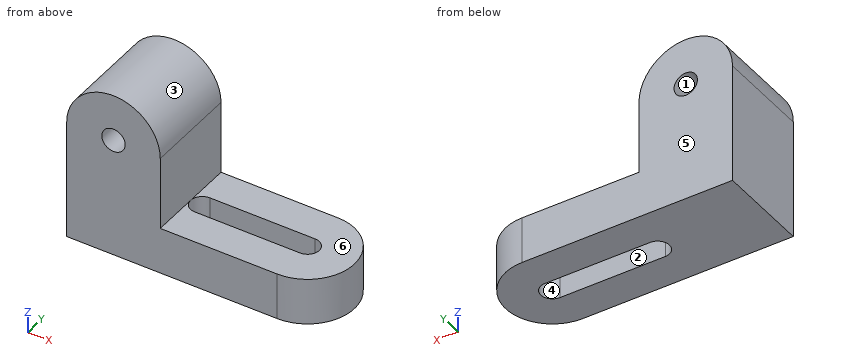
```python
from build123d import *

# Parameters (mm, degrees)
F1_DEPTH = 50.8
F2_R     = 12.7
F3_DEPTH = 101.6


with BuildPart() as f1:
    # F0 (on Top) → F1 (new body)
    with BuildSketch(Plane.XY):
        with BuildLine():
            ThreePointArc((114.3, -50.8), (165.1, 0), (114.3, 50.8))
            Line((114.3, 50.8), (-114.3, 50.8))
            Line((-114.3, 50.8), (-114.3, -50.8))
            Line((-114.3, -50.8), (114.3, -50.8))
        make_face()
        with BuildLine():
            Line((114.3, -12.7), (0, -12.7))
            ThreePointArc((0, -12.7), (-12.7, 0), (0, 12.7))
            Line((0, 12.7), (114.3, 12.7))
            ThreePointArc((114.3, 12.7), (127, 0), (114.3, -12.7))
        make_face(mode=Mode.SUBTRACT)
    extrude(amount=F1_DEPTH)

    # F2 (on face) → F3 (join)
    with BuildSketch(Plane.XZ.offset(50.8)):
        with BuildLine():
            Line((-114.3, 50.8), (-12.7, 50.8))
            Line((-12.7, 50.8), (-12.7, 130.381152))
            ThreePointArc((-12.7, 130.381152), (-63.5, 181.181152), (-114.3, 130.381152))
            Line((-114.3, 130.381152), (-114.3, 50.8))
        make_face()
        with Locations((-63.5, 130.381152)):
            Circle(F2_R, mode=Mode.SUBTRACT)
    extrude(amount=-F3_DEPTH)


solid = f1.part
```
Model file for the job. Use its own axes, mm. Face numbers are marked on the shaded views. A direction names the side the tool comes from. Give positions to 0.01 mm unless a question says otherwise; leave off trailing zeros. Loops run counter-clockwise (first coordinate to the right, second up) from the corner with the lowest first, then second, coordinate; pieces in that order, holes last. Notation, with made-up numbers: (43.5, 38) -> (75.5, 38) arc R13 cw to (75.5, 63) -> close; hole circle Ø7 at (-14, -27). An arc over 180 degrees is marked (long way). Use CSV: the item, a comma, the result in double quotes. Start each with the question number.
1) Wall check: line 1 (Z direction, x = -63.5, y = 23); line 2 (Y direction, x = 55.5, z = 40); line 3 (X direction, y = -26, z = 99). Give the ranges that are in metal, low to high.
2) Slice it at A-A on x = 78.5. Give the cut face in (y, z).
3) Tool access for the marked faces 4, 5 and 6: list every direction of +Z, -Z, +X, -X, +Y, -Y with a clear straight run to the whole face (end or side of a thin tool).
4) Slice it at D-D on y = 32. Give the cut face in (x, z).
5) Slice it at B-B on z = 124. Give the cut face in (x, y), plus the area to 3 significant figures.
6) Mould opens along Z. For the marked faces 1, 2 and 3 say: released by +Z, released by -Z, zero draft, split by the parting line, or undercut.
7) Slice it at C-C on y = -9. Give the cut face in (x, z), plus the area to 3 significant figures.
8) Flat gauge pins, fed straight in: pin 1 Ø3 at (x, z) = (131, 41) entering from +Y; pin 2 Ø8 at (y, z) = (15, 141) entering from +X; pin 3 Ø12 at (y, z) = (0.5, 149) entering from +X; pin 4 Ø23 at (x, z) = (-63.5, 130.38) entering from -Y. Where does each tip first touch, or does it go through?
Computed values:
1,line 1,"z = 0 to 117.68, 143.08 to 181.18"
1,line 2,"y = -50.8 to -12.7, 12.7 to 50.8"
1,line 3,"x = -114.3 to -12.7"
2,outline,"(-50.8, 0) -> (-12.7, 0) -> (-12.7, 50.8) -> (-50.8, 50.8) -> close; (12.7, 0) -> (50.8, 0) -> (50.8, 50.8) -> (12.7, 50.8) -> close"
3,face 4,"+Z, -Z"
3,face 5,"+Z, -Z, +X, -X, +Y"
3,face 6,"+Z, +X, +Y, -Y"
4,outline,"(-114.3, 0) -> (153.75, 0) -> (153.75, 50.8) -> (-12.7, 50.8) -> (-12.7, 130.38) arc R50.8 ccw to (-114.3, 130.38) -> close; hole circle Ø25.4 at (-63.5, 130.38)"
5,outline,"(-114.3, -50.8) -> (-74.48, -50.8) -> (-74.48, 50.8) -> (-114.3, 50.8) -> close; (-52.52, -50.8) -> (-12.7, -50.8) -> (-12.7, 50.8) -> (-52.52, 50.8) -> close"
5,area,"8,090 mm^2"
6,face 1,"undercut"
6,face 2,"zero draft"
6,face 3,"released by +Z"
7,outline,"(-114.3, 0) -> (-8.96, 0) -> (-8.96, 50.8) -> (-12.7, 50.8) -> (-12.7, 130.38) arc R50.8 ccw to (-114.3, 130.38) -> close; (123.26, 0) -> (164.3, 0) -> (164.3, 50.8) -> (123.26, 50.8) -> close; hole circle Ø25.4 at (-63.5, 130.38)"
7,area,"19,100 mm^2"
8,pin 1,"stops at y = 48.47"
8,pin 2,"stops at x = -13.13"
8,pin 3,"stops at x = -14.29"
8,pin 4,"passes through"
